Build history of the part. All positions in model axes, mm. A direction names the side the tool comes from. Give positions to 0.01 mm unless a question says otherwise; leave off trailing zeros. Loops run counter-clockwise (first coordinate to the right, second up) from the corner with the lowest first, then second, coordinate; pieces in that order, holes last. Notation, with made-up numbers: (-13, 59.25) -> (7, 59.25) arc R13 cw to (7, 63.25) -> close; hole circle Ø2 at (-23, -36). An arc over 180 degrees is marked (long way). Answer in a Markdown table with one row per item. Add a question column.
Autodesk Inventor part; units mm, degrees
ref_plane "YZ Plane" through (0, 0, 0) normal (1, 0, 0) x (0, 1, 0)
ref_plane "XZ Plane" through (0, 0, 0) normal (0, 1, 0) x (-1, 0, 0)
ref_plane "XY Plane" through (0, 0, 0) normal (0, 0, 1) x (1, 0, 0)
sketch "Sketch1" plane through (0, 0, 0) normal (0, 1, 0) x (-1, 0, 0)
  line L0 (-24.55, -31.25) -> (24.55, -31.25)
  line L1 (24.55, -31.25) -> (24.55, 31.25)
  line L2 (24.55, 31.25) -> (-24.55, 31.25)
  line L3 (-24.55, 31.25) -> (-24.55, -31.25)
  line L4 (-24.55, -31.25) -> (24.55, 31.25) construction
  line L5 (24.55, -31.25) -> (-24.55, 31.25) construction
  point P0 (0, 0)
  dimension "d0" = 62.5
  dimension "d1" = 49.1
extrude "Extrusion1" add sketch "Sketch1" along normal blind 6
sketch "Sketch2" plane through (0, 6, 0) normal (0, 1, 0) x (1, 0, 0)
  line L0 (22.55, 29.25) -> (-22.55, 29.25)
  line L1 (-22.55, 29.25) -> (-22.55, -29.25)
  line L2 (-22.55, -29.25) -> (22.55, -29.25)
  line L3 (22.55, -29.25) -> (22.55, 29.25)
  line L4 (22.55, 29.25) -> (-22.55, -29.25) construction
  line L5 (-22.55, 29.25) -> (22.55, -29.25) construction
  line L6 (-24.55, 31.25) -> (-24.55, -31.25)
  line L7 (-24.55, -31.25) -> (24.55, -31.25)
  arc A0 (-22.55, -28.25) -> (-21.55, -29.25) centre (-22.55, -29.25) ccw
  arc A1 (21.55, -29.25) -> (22.55, -28.25) centre (22.55, -29.25) ccw
  arc A2 (-21.55, 29.25) -> (-22.55, 28.25) centre (-22.55, 29.25) ccw
  arc A3 (22.55, 28.25) -> (21.55, 29.25) centre (22.55, 29.25) ccw
  point P0 (0, 0)
  dimension "d4" = 2
  dimension "d5" = 2
  dimension "d32" = 1
  dimension "d33" = 1
  dimension "d34" = 1
  dimension "d35" = 1
extrude "Extrusion2" cut sketch "Sketch2" against normal blind 0.5
sketch "Sketch3" plane through (0, 5.5, 0) normal (0, 1, 0) x (1, 0, 0)
  line L0 (-22.55, -28.25) -> (-22.55, 28.25)
  line L1 (22.55, 28.25) -> (-22.55, 28.25)
  line L2 (-22.55, 28.25) -> (-22.55, -28.25)
  line L3 (-22.55, -28.25) -> (22.55, -28.25)
  line L4 (22.55, -28.25) -> (22.55, 28.25)
  line L5 (22.55, 28.25) -> (-22.55, -28.25) construction
  line L6 (-22.55, 28.25) -> (22.55, -28.25) construction
  line L7 (21.55, -29.25) -> (-21.55, -29.25)
  point P0 (0, 0)
  point P1 (-22.3, -29)
  point P2 (-22.3, 29)
  point P3 (22.3, -29)
  point P4 (-22.3, 28)
  point P5 (-21.55, -29.25)
  dimension "d8" = 1
extrude "Extrusion3" cut sketch "Sketch3" against normal blind 3.5
sketch "Sketch8" plane through (0, 2, 0) normal (0, 1, 0) x (1, 0, 0)
  line L0 (-20.25, -14.25) -> (20.25, -14.25)
  line L1 (20.25, -14.25) -> (20.25, 14.25)
  line L2 (20.25, 14.25) -> (-20.25, 14.25)
  line L3 (-20.25, 14.25) -> (-20.25, -14.25)
  line L4 (-20.25, -14.25) -> (20.25, 14.25) construction
  line L5 (20.25, -14.25) -> (-20.25, 14.25) construction
  point P0 (0, 0)
  dimension "d28" = 28.5
  dimension "d29" = 40.5
extrude "Extrusion6" cut sketch "Sketch8" against normal through all
sketch "Sketch9" plane through (0, 6, 0) normal (0, 1, 0) x (1, 0, 0)
  line L0 (24.55, -28.25) -> (-24.55, -28.25)
  line L1 (-24.55, -28.25) -> (-24.55, -31.25)
  line L2 (-24.55, -31.25) -> (24.55, -31.25)
  line L3 (24.55, -31.25) -> (24.55, -28.25)
  line L4 (24.55, -31.25) -> (24.55, 31.25)
  line L5 (-21.55, 29.25) -> (21.55, 29.25)
  point P0 (0, 0)
  dimension "d36" = 57.5
extrude "Extrusion7" cut sketch "Sketch9" against normal through all
sketch "Sketch10" plane through (0, 2, 0) normal (0, 1, 0) x (1, 0, 0)
  line L0 (22.55, -28.25) -> (-22.55, -28.25)
  line L1 (-22.55, -28.25) -> (22.55, -28.25)
  line L2 (22.55, -28.25) -> (22.55, -27.25)
  line L3 (22.55, -27.25) -> (-22.55, -27.25)
  line L4 (-22.55, -27.25) -> (-22.55, -28.25)
  point P0 (0, 0)
  dimension "d39" = 1
extrude "Extrusion8" add sketch "Sketch10" along normal up to surface (3.5 mm away)
equation "\"d5\" = d4"
equation "\"d33\" = d32"
equation "\"d34\" = d32"
equation "\"d35\" = d32"
properties part number "Module Cover" material "ABS Plastic"
(1) Saw through at B-B, the plane y = 1. List the corners of the cut face in (x, z), then the cut area to 3 significant figures.
(2) 3-axis set-ups, long thin cutter, end or side, ignore diameter. For faces 1 (the cylindrical face through (-23.233, 5.754, -29.98)), 2 (the flat face through (0, 1, -14.25)), 3 (the flat face through (0, 0, -21)): which of +Z, -Z, +X, -X, +Y, -Y reach the whole face in a straight line?
(3) Saw through at A-A, the plane x = -6.5. List the corners of the cut face in (y, z), then the cut area to 3 significant figures.
(4) Two-plate mould, pull along X, no slides. Class faces 4 (the flat face through (-24.55, 3, -2)), 5 (the flat face through (0, 6, -30)), 6 (the flat face through (0, 4, 27.25)): released by +X, released by -X, zero draft, split by the parting line, or undercut.
(5) Flat gauge pin, fed straight in: pin 1 Ø1.1 at (x, z) = (-3, 28) entering from +Y. Where does the tip first touch, or does it go through?
(6) Saw through at D-D, the plane y = 4.1. List the corners of the cut face in (x, z).
(7) Wall check: line 1 along X through (y, z) = (2.6, -20.5); line 2 along Z through (x, y) = (-19, 4.7); line 3 along X through (y, z) = (1.1, -2.5). Give the ranges that are in metal, low to high. Write a range as from..to.
(8) Saw through at C-C, the plane z = -20.5. List the corners of the cut face in (x, y), then the cut area to 3 significant figures.
Worked answers:
| question | item | result |
|---|---|---|
| 1 | outline | (-24.55, -31.25) -> (24.55, -31.25) -> (24.55, 28.25) -> (-24.55, 28.25) -> close; hole (-20.25, -14.25) -> (20.25, -14.25) -> (20.25, 14.25) -> (-20.25, 14.25) -> close |
| 1 | area | 1,770 mm^2 |
| 2 | face 1 | +Y |
| 2 | face 2 | +Y, -Y |
| 2 | face 3 | +Z, -Z, +X, -X, -Y |
| 3 | outline | (0, -31.25) -> (6, -31.25) -> (6, -29.25) -> (5.5, -29.25) -> (5.5, -28.25) -> (2, -28.25) -> (2, -14.25) -> (0, -14.25) -> close; (0, 14.25) -> (2, 14.25) -> (2, 27.25) -> (5.5, 27.25) -> (5.5, 28.25) -> (0, 28.25) -> close |
| 3 | area | 77.0 mm^2 |
| 4 | face 4 | released by -X |
| 4 | face 5 | zero draft |
| 4 | face 6 | undercut |
| 5 | pin 1 | y = 5.5 |
| 6 | outline | (-24.55, -31.25) -> (24.55, -31.25) -> (24.55, 28.25) -> (-24.55, 28.25) -> close; hole (-22.55, -28.25) -> (22.55, -28.25) -> (22.55, 27.25) -> (-22.55, 27.25) -> close |
| 7 | line 1 | -24.55..-22.55, 22.55..24.55 |
| 7 | line 2 | -31.25..-28.25, 27.25..28.25 |
| 7 | line 3 | -24.55..-20.25, 20.25..24.55 |
| 8 | outline | (-24.55, 0) -> (24.55, 0) -> (24.55, 6) -> (22.55, 6) -> (22.55, 2) -> (-22.55, 2) -> (-22.55, 6) -> (-24.55, 6) -> close |
| 8 | area | 114 mm^2 |
